Input: part model. Units: mm. Frame: model coordinates. Round coordinates to 2 decimals unless told otherwise and drop trailing zeros. Write each loop counter-clockwise with the first axis right and the second up, starting at its lowest first coordinate (ties: lowest second). Pieces come first, ordered by that corner, then holes. Notation, with made-up numbers: (15.5, -8.5) - (71.5, -8.5) arc R13 ccw to (71.5, 13.5) - close; hole circle Ø8 at (-5, -26). An arc over 180 degrees is marked (long way). One line per item, written item: value. Start each with the question number.
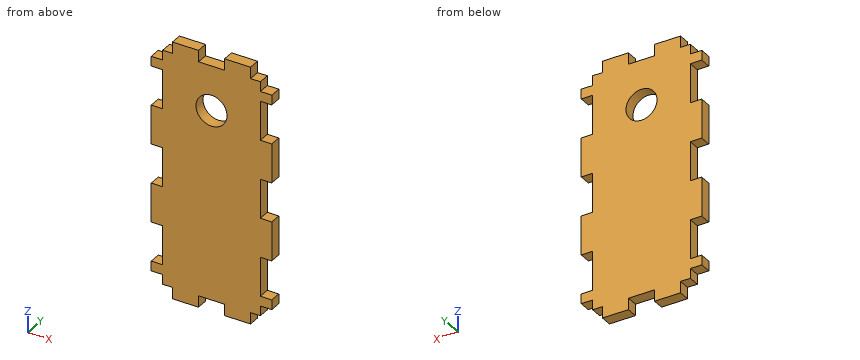
```python
from build123d import *

# Parameters (mm, degrees)
F0_R     = 7.9375
F0_W     = 13.333333
F0_H     = 5.842
F0_W_2   = 5.842
F0_H_2   = 5
F0_H_3   = 20
F1_DEPTH = 5.842


with BuildPart() as f1:
    # F0 (on Front) → F1 (new body)
    with BuildSketch(Plane.XZ):
        Polygon((-20, 60), (-25, 60), (-25, 55), (-25, 50), (-25, 30), (-25, 10), (-25, -10), (-25, -30), (-25, -50), (-25, -55), (-25, -60), (-20, -60), (-6.666667, -60), (6.666667, -60), (20, -60), (25, -60), (25, -55), (25, -50), (25, -30), (25, -10), (25, 10), (25, 30), (25, 50), (25, 55), (25, 60), (20, 60), (6.666667, 60), (-6.666667, 60), align=None)
        with Locations((0, 37.0625)):
            Circle(F0_R, mode=Mode.SUBTRACT)
        with Locations((-13.333334, 62.921)):
            Rectangle(F0_W, F0_H)
        with Locations((-27.921, 52.5)):
            Rectangle(F0_W_2, F0_H_2)
        with Locations((13.333334, 62.921)):
            Rectangle(F0_W, F0_H)
        with Locations((-27.921, 20)):
            Rectangle(F0_W_2, F0_H_3)
        with Locations((-27.921, -20)):
            Rectangle(F0_W_2, F0_H_3)
        with Locations((27.921, 52.5)):
            Rectangle(F0_W_2, F0_H_2)
        with Locations((-27.921, -52.5)):
            Rectangle(F0_W_2, F0_H_2)
        with Locations((27.921, 20)):
            Rectangle(F0_W_2, F0_H_3)
        with Locations((27.921, -20)):
            Rectangle(F0_W_2, F0_H_3)
        with Locations((-13.333334, -62.921)):
            Rectangle(F0_W, F0_H)
        with Locations((27.921, -52.5)):
            Rectangle(F0_W_2, F0_H_2)
        with Locations((13.333334, -62.921)):
            Rectangle(F0_W, F0_H)
    extrude(amount=F1_DEPTH)


solid = f1.part
```
Q1. Cut plane B-B, the plane z = -42.5. Output: boundary loops of the cut face in (x, y), and give its area (3 significant figures).
Q2. Contact query for flat-ended pins moving along their axis: pin 1 Ø3 at (x, y) = (-28, -2.5) entering from -Z; pin 2 Ø3 at (y, z) = (-4, -63) entering from -X; pin 3 Ø2 at (y, z) = (-2, 1) entering from -X. Output: stop coordinate, or through.
Q3. Cut plane A-A, the plane x = 0. Output: boundary loops of the cut face in (y, z) (3 decimals), and give its area (3 significant figures).
Q4. Material intervals for probe 1 along X at (y, z) = (-1.65, -30.5); probe 2 along X at (y, z) = (-4.75, 41.5); probe 3 along X at (y, z) = (-4.4, 39), sorted ascending. Write a range as from..to.
A:
1. outline: (-25, -5.84) - (25, -5.84) - (25, 0) - (-25, 0) - close
1. area: 292 mm²
2. pin 1: stops at z = -55
2. pin 2: stops at x = -20
2. pin 3: stops at x = -25
3. outline: (-5.842, -60) - (0, -60) - (0, 29.125) - (-5.842, 29.125) - close; (-5.842, 45) - (0, 45) - (0, 60) - (-5.842, 60) - close
3. area: 608 mm²
4. probe 1: x = -25..25
4. probe 2: x = -25..-6.58, 6.58..25
4. probe 3: x = -25..-7.7, 7.7..25
